Autodesk Inventor part; units mm, degrees
ref_plane "YZ Plane" through (0, 0, 0) normal (1, 0, 0) x (0, 1, 0)
ref_plane "XZ Plane" through (0, 0, 0) normal (0, 1, 0) x (-1, 0, 0)
ref_plane "XY Plane" through (0, 0, 0) normal (0, 0, 1) x (1, 0, 0)
sketch "スケッチ1" plane through (0, 0, 0) normal (0, 1, 0) x (-1, 0, 0)
  circle A0 centre (0, 0) radius 20
  dimension "d0" = 40
extrude "押し出し1" add sketch "スケッチ1" along normal blind 58.7
sketch "スケッチ2" plane through (0, 58.7, 0) normal (0, 1, 0) x (1, 0, 0)
  circle A0 centre (0, 0) radius 12
  dimension "d3" = 24
extrude "押し出し2" add sketch "スケッチ2" along normal blind 3
hole "穴1" at (11.3305, 58.7, -10.9462) direction (0, -1, 0) diameter 4 depth 7
hole "穴2" at (-10.866, 58.7, 12.1709) direction (0, -1, 0) diameter 4 depth 7
hole "穴3" at (-11.4749, 58.7, -10.9538) direction (0, -1, 0) diameter 4 depth 7
hole "穴4" at (11.3606, 58.7, 10.8461) direction (0, -1, 0) diameter 4 depth 7
properties part number "HarmonicDrive1"
Input: part model. Units: mm. Frame: model coordinates. A direction names the side the tool comes from. Coordinates: 2 decimals unless noted, no trailing zeros. Loops run counter-clockwise (first coordinate to the right, second up) from the corner with the lowest first, then second, coordinate; pieces in that order, holes last. Notation, with made-up numbers: M -12.75,-38.5 L -3.75,-38.5 A24 ccw -3.75,-2.5 Z; hole C 41,65 d4. An arc over 180 degrees is marked long. Use a Markdown table: item, result. Add a question column.
1) Pin query (flat end, axial travel): P1, Ø4.5, axis at x = 11.36, z = 10.85, coming from the -Y side; P2, Ø4, axis at x = -8.5, y = 26.5, coming from the -Z side; P3, Ø1.5, axis at y = 48.5, z = 1, coming from the -X side; P4, Ø1.2, axis at x = -11, z = -10, coming from the +Y side. Return the tip coordinate at first contact, or that it passes through.
2) Section C-C, the plane y = 58. Return the cut outline in (x, z), plus the area to 3 significant figures.
3) Section D-D, the plane y = 28. Return the cut outline in (x, z).
4) Set-up query: faces 1 (the flat face through (-9, 58.7, -9)), 2 (the flat face through (0, 0, 0)). Return all of +Z, -Z, +X, -X, +Y, -Y with unobstructed straight access to the full face (end or side cutting, diameter ignored); none if empty.
5) Section A-A, the plane z = 0. Return the cut outline in (x, y).
6) Line query: L1, parallel to Y at x = 9.5, z = 10; L2, parallel to Y at x = 11, z = 10; L3, parallel to Z at x = -14, y = 29. Output: solid intervals per line, ascending. Write a range as from..to.
7) Draft query along Z for faces 3 (the cylindrical face through (4.336, 28.939, 19.524)), 4 (the flat face through (-11, 51.7, 12)), 5 (the flat face through (0, 61.7, 0)). Return one class per face: +Z half, -Z half, draft (parallel to the pull), parting line (faces both ways), or undercut.
8) Section B-B, the plane x = 0. Return the cut outline in (y, z).
Answer below:
| question | item | result |
|---|---|---|
| 1 | P1 | y = 0 |
| 1 | P2 | z = -18.91 |
| 1 | P3 | x = -20 |
| 1 | P4 | y = 51.7 |
| 2 | outline | C 0,0 d40; hole C -11.47,-10.95 d4; hole C -10.87,12.17 d4; hole C 11.33,-10.95 d4; hole C 11.36,10.85 d4 |
| 2 | area | 1,210 mm2 |
| 3 | outline | C 0,0 d40 |
| 4 | face 1 | +Y |
| 4 | face 2 | +Z, -Z, +X, -X, -Y |
| 5 | outline | M -20,0 L 20,0 L 20,58.7 L 12,58.7 L 12,61.7 L -12,61.7 L -12,58.7 L -20,58.7 Z |
| 6 | L1 | 0..58.7 |
| 6 | L2 | 0..51.7 |
| 6 | L3 | -14.28..14.28 |
| 7 | face 3 | parting line |
| 7 | face 4 | undercut |
| 7 | face 5 | draft |
| 8 | outline | M 0,-20 L 58.7,-20 L 58.7,-12 L 61.7,-12 L 61.7,12 L 58.7,12 L 58.7,20 L 0,20 Z |
